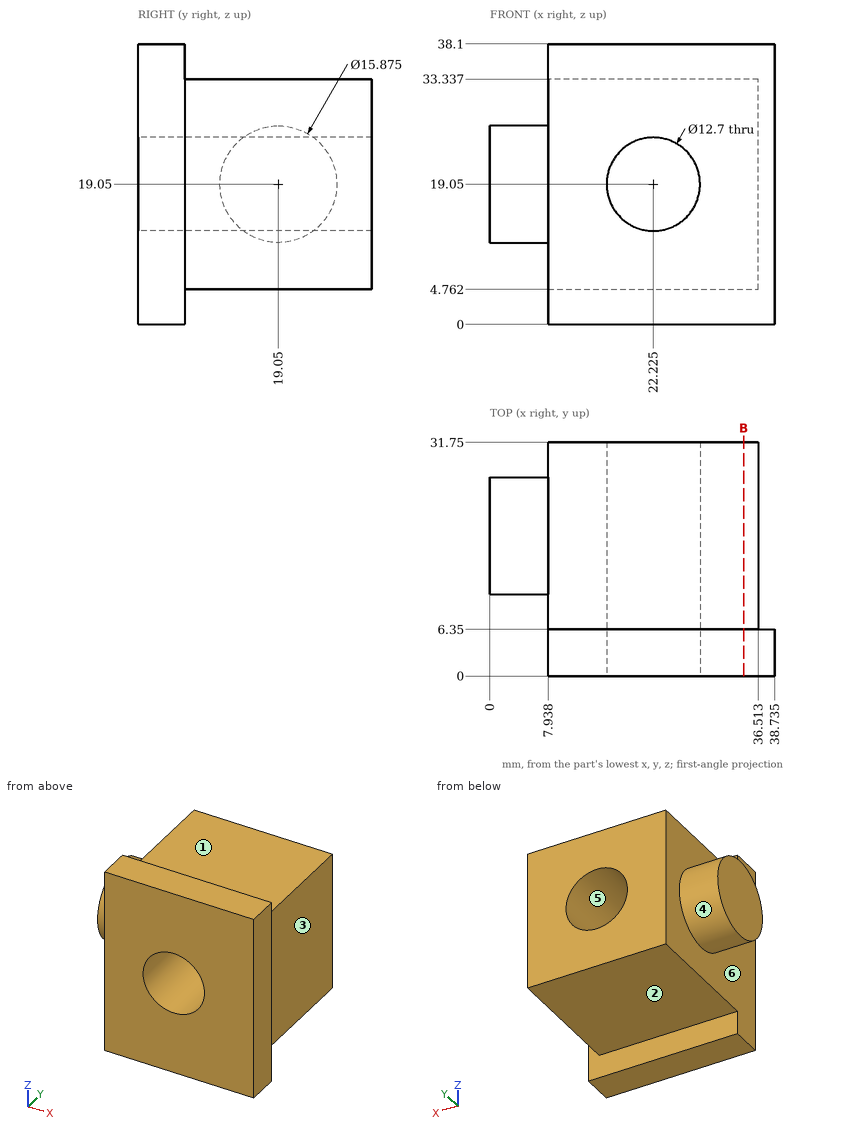
Here's the drawing with two shaded views (mm, measured from the low corner). I have some questions. A direction names the side the tool comes from. Coordinates: 2 decimals unless noted, no trailing zeros. Order: outer loops, then holes, each group sorted by start corner. A loop starts at its lowest first (then second) coordinate and runs counter-clockwise, first axis right, second up.
Q1. Suppose I cut it at B-B on x = 34.5. Please give me the cut outline in (y, z).
Q2. Which directions (+Z, -Z, +X, -X, +Y, -Y) give clear straight access to the entire face, cutting with the end or side of a thin tool? Please do the marked faces 1, 2 and 3.
Q3. Thinking about a two-plate mould opening in X: for the marked faces 4, 5 and 6, which applies, released by +X, released by -X, zero draft, split by the parting line, or undercut?
Q4. Will these pins go through, and if not, where does the flat tip stop? pin 1 (12.5 mm diameter, centred on x = 22.5, y = 23.5, fed in from -Z); pin 2 (1.5 mm diameter, centred on y = 4.5, z = 16, fed in from -X); pin 3 (4 mm diameter, centred on y = 23, z = 23.5, fed in from +X).
Q5. Please list where these lines run through material, in increasing order: L1, parallel to X at y = 15, z = 19.05 (1 decimal); L2, parallel to X at y = 10, z = 19.05 (1 decimal); L3, parallel to X at y = 7, z = 28.
Answer:
1. outline: (0, 0) - (6.35, 0) - (6.35, 4.76) - (31.75, 4.76) - (31.75, 33.34) - (6.35, 33.34) - (6.35, 38.1) - (0, 38.1) - close
2. face 1: +Z, +X, -X, +Y
2. face 2: -Z, +X, -X, +Y
2. face 3: +Z, -Z, +X, +Y
3. face 4: zero draft
3. face 5: undercut
3. face 6: released by -X
4. pin 1: stops at z = 4.76
4. pin 2: stops at x = 7.94
4. pin 3: stops at x = 36.51
5. L1: x = 0 to 15.9, 28.6 to 36.5
5. L2: x = 7.9 to 15.9, 28.6 to 36.5
5. L3: x = 7.94 to 36.51
